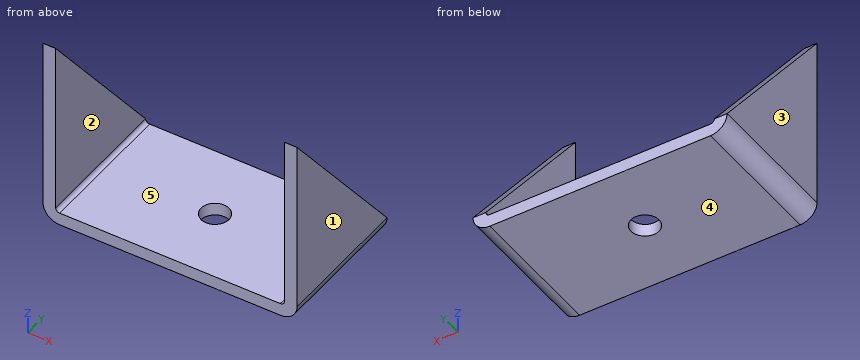
from build123d import *

# Parameters (mm, degrees)
SKETCH2_W                    = 57.15
SKETCH2_H                    = 34.925
BASE_FLANGE1_DEPTH           = 3.175
EDGE_FLANGE1_STRIP_W         = 14.7
EDGE_FLANGE1_STRIP_H         = 3.175
EDGE_FLANGE1_STRIP_CUT_DEPTH = 34.925
EDGE_FLANGE1_DEPTH           = 34.925
CUT_EXTRUDE1_DEPTH           = 3.175
M6_CLEARANCE_HOLE1_D         = 7


# Sheet-metal steps are written as plain solids
with BuildPart() as part:
    # Sketch2 → Base-Flange1 (new body)
    with BuildSketch(Plane.XY):
        Rectangle(SKETCH2_W, SKETCH2_H)
    extrude(amount=BASE_FLANGE1_DEPTH)

    # Edge-Flange1 strip (across the edge) → Edge-Flange1 strip cut (cut)
    with BuildSketch(Plane(origin=(28.575, -17.4625, 3.175), x_dir=(-1, 0, 0), z_dir=(0, 1, 0))):
        with Locations((-6.35, -1.5875)):
            Rectangle(EDGE_FLANGE1_STRIP_W, EDGE_FLANGE1_STRIP_H)
    edge_flange1_strip_cut = extrude(amount=EDGE_FLANGE1_STRIP_CUT_DEPTH, mode=Mode.SUBTRACT)

    # Edge-Flange1 section (across the edge) → Edge-Flange1 (add)
    with BuildSketch(Plane(origin=(28.575, -17.4625, 3.175), x_dir=(-1, 0, 0), z_dir=(0, 1, 0))):
        with BuildLine():
            Line((-3.175, 1), (-3.175, 44.45))
            Line((-3.175, 44.45), (0, 44.45))
            Line((0, 44.45), (0, 1))
            ThreePointArc((0, 1), (0.292893219, 0.292893219), (1, 0))
            Line((1, 0), (1, -3.175))
            ThreePointArc((1, -3.175), (-1.952170811, -1.952170811), (-3.175, 1))
        make_face()
    edge_flange1 = extrude(amount=EDGE_FLANGE1_DEPTH)

    # Sketch10 → Cut-Extrude1 (cut)
    with BuildSketch(Plane(origin=(31.75, 0, 0), x_dir=(0, 0, -1), z_dir=(1, 0, 0))):
        Polygon((-4.175, 17.4625), (-47.625, -17.4625), (-47.625, 17.4625), align=None)
    cut_extrude1 = extrude(amount=-CUT_EXTRUDE1_DEPTH, mode=Mode.SUBTRACT)

    # Mirror1: Edge-Flange1 strip cut, Edge-Flange1, Cut-Extrude1 across plane
    add(edge_flange1_strip_cut.mirror(Plane(origin=(0, 0, 0), x_dir=(0, 0, 1), z_dir=(1, 0, 0))), mode=Mode.SUBTRACT)
    add(edge_flange1.mirror(Plane(origin=(0, 0, 0), x_dir=(0, 0, 1), z_dir=(1, 0, 0))))
    add(cut_extrude1.mirror(Plane(origin=(0, 0, 0), x_dir=(0, 0, 1), z_dir=(1, 0, 0))), mode=Mode.SUBTRACT)

    # M6 Clearance Hole1 (through all)
    with Locations(Plane.XY.offset(3.175)):
        with Locations((0, 0)):
            Hole(M6_CLEARANCE_HOLE1_D / 2)


solid = part.part
Geometry: final body of the model. Coordinates: model frame, mm. Face numbers are marked on the shaded views. A direction names the side the tool comes from. Give positions to 0.01 mm unless a question says otherwise; leave off trailing zeros. Loops run counter-clockwise (first coordinate to the right, second up) from the corner with the lowest first, then second, coordinate; pieces in that order, holes last. Notation, with made-up numbers: (77.25, 1.25) - (83.25, 1.25) arc R28 cw to (83.25, 30.25) - close; hole circle Ø5 at (46, 27.25). An arc over 180 degrees is marked (long way). Answer as CSV lines item,"result". Start each with the question number.
1. Section C-C, the plane x = 0. Return loops of the section in (y, z) (1 decimal).
2. Ray query, L1, parallel to X at y = -3.5, z = 27 (3 decimals); L2, parallel to Y at x = 0, z = 2.35; L3, parallel to Z at x = 19.5, y = 2 (3 decimals). Return the intervals inside material, ascending.
3. Section A-A, the plane y = 0. Return loops of the section in (x, z) (3 decimals).
4. Reachability of the marked faces 4 and 5 from +Z, -Z, +X, -X, +Y, -Y: full face, straight path, thin tool, end or side. Return the list, or none.
5. Section D-D, the plane y = -10.5. Return loops of the section in (x, z) (3 decimals), plus the area to 3 significant figures.
6. Draft query along X for the marked faces 1, 2 and 3. Return one class per face: released by +X, released by -X, zero draft, split by the parting line, or undercut.
Answers:
1,outline,"(-17.5, 0) - (-3.5, 0) - (-3.5, 3.2) - (-17.5, 3.2) - close; (3.5, 0) - (17.5, 0) - (17.5, 3.2) - (3.5, 3.2) - close"
2,L1,"x = -31.75 to -28.575, 28.575 to 31.75"
2,L2,"y = -17.46 to -3.5, 3.5 to 17.46"
2,L3,"z = 0 to 3.175"
3,outline,"(-31.75, 4.175) arc R4.175 ccw to (-27.575, 0) - (-3.5, 0) - (-3.5, 3.175) - (-27.575, 3.175) arc R1 cw to (-28.575, 4.175) - (-28.575, 25.9) - (-31.75, 25.9) - close; (3.5, 0) - (27.575, 0) arc R4.175 ccw to (31.75, 4.175) - (31.75, 25.9) - (28.575, 25.9) - (28.575, 4.175) arc R1 cw to (27.575, 3.175) - (3.5, 3.175) - close"
4,face 4,"-Z, +X, -X, +Y, -Y"
4,face 5,"+Z, +Y, -Y"
5,outline,"(-31.75, 4.175) arc R4.175 ccw to (-27.575, 0) - (27.575, 0) arc R4.175 ccw to (31.75, 4.175) - (31.75, 38.963) - (28.575, 38.963) - (28.575, 4.175) arc R1 cw to (27.575, 3.175) - (-27.575, 3.175) arc R1 cw to (-28.575, 4.175) - (-28.575, 38.963) - (-31.75, 38.963) - close"
5,area,"422 mm2"
6,face 1,"released by +X"
6,face 2,"undercut"
6,face 3,"released by -X"
